Can you work these out from the model? Positions are in its coordinate system, mm. Face numbers are marked on the shaded views. A direction names the side the tool comes from. Round coordinates to 2 decimals unless told otherwise and drop trailing zeros. Write each loop counter-clockwise with the first axis right and the second up, starting at its lowest first coordinate (ties: lowest second). Pieces come first, ordered by that corner, then holes. Notation, with made-up numbers: M 47,8 L 64,8 A28 ccw 64,36 Z; hole C 8,68 d9. An arc over 180 degrees is marked long. Answer in a Markdown table with one row per item. Add a question column.
(1) If I drill on probe 1 along X at (y, z) = (-2.75, 6.2); probe 2 along Z at (x, y) = (29.2, 18.25); probe 3 along X at (y, z) = (36, 5.5), over which ranges is the centre line in solid material (lowest first)?
(2) If we mould it in two halves opening along X, with no side actions, what happens to the marked faces 1, 2, 3 and 4? For each: released by +X, released by -X, zero draft, split by the parting line, or undercut.
(3) I'm going to push flat-ended pins straight in: pin 1 (3.5 mm diameter, centred on x = 32.5, z = 12.5, fed in from -Y); pin 2 (2 mm diameter, centred on x = 5, z = 7, fed in from +Y); pin 3 (3 mm diameter, centred on y = 17.5, z = 10.5, fed in from -X). Where does each tip first touch, or does it pass through?
(4) For the marked faces 5, 6 and 7, which set-ups out of +Z, -Z, +X, -X, +Y, -Y let a thin tool reach every point of the face, with its end or its side?
(5) Suppose I cut it at A-A, the plane y = 18.25. Write out the boundary of the cut face in (x, z), then the cut area to 3 significant figures.
(6) Suppose I cut it at B-B, the plane z = 6.2. Write out the boundary of the cut face in (x, y), then the cut area to 3 significant figures.
(7) Suppose I cut it at D-D, the plane x = 16.5. Write out the boundary of the cut face in (y, z), then the cut area to 3 significant figures.
(8) Suppose I cut it at C-C, the plane z = 2.5. Write out the boundary of the cut face in (x, y).
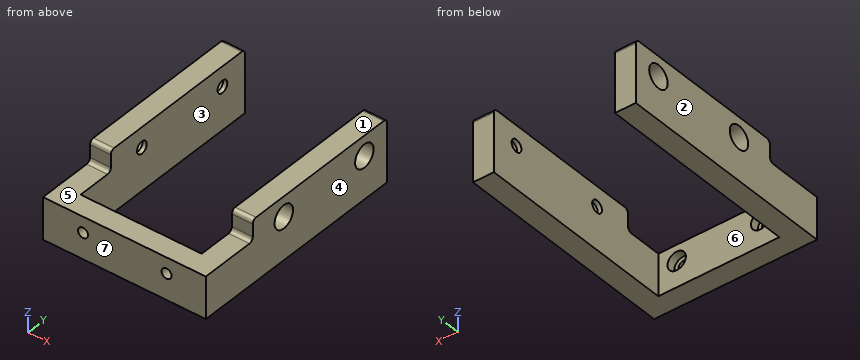
from build123d import *

# Parameters (mm, degrees)
BOSS_EXTRUDE1_DEPTH              = 10
SKETCH2_W                        = 5
SKETCH2_H                        = 40
BOSS_EXTRUDE2_DEPTH              = 5
CBORE_FOR_M2_SHCS1_D             = 2.4
CBORE_FOR_M2_SHCS1_CBORE_D       = 4.4
CBORE_FOR_M2_SHCS1_CBORE_DEPTH   = 2
CBORE_FOR_M2_5_SHCS1_D           = 2.9
CBORE_FOR_M2_5_SHCS1_DEPTH       = 5
CBORE_FOR_M2_5_SHCS1_CBORE_D     = 5.5
CBORE_FOR_M2_5_SHCS1_CBORE_DEPTH = 4
CBORE_FOR_M2_5_SHCS2_D           = 2.9
CBORE_FOR_M2_5_SHCS2_CBORE_D     = 5.5
CBORE_FOR_M2_5_SHCS2_CBORE_DEPTH = 4
FILLET1_R                        = 1


with BuildPart() as part:
    # Sketch1 → Boss-Extrude1 (new body)
    with BuildSketch(Plane.XY):
        Polygon((0, 0), (0, 49), (-5, 49), (-5, -5), (34, -5), (34, 49), (29, 49), (29, 0), align=None)
    extrude(amount=BOSS_EXTRUDE1_DEPTH)

    # Sketch2 → Boss-Extrude2 (add)
    with BuildSketch(Plane.XY.offset(10)):
        with Locations((-2.5, 29)):
            Rectangle(SKETCH2_W, SKETCH2_H)
    boss_extrude2 = extrude(amount=BOSS_EXTRUDE2_DEPTH)

    # Mirror1: Boss-Extrude2 across plane
    add(boss_extrude2.mirror(Plane.ZY.offset(-14.5)))

    # CBORE for M2 SHCS1 (through all)
    with Locations(Plane(origin=(0, 0, 0), x_dir=(1, 0, 0), z_dir=(0, 1, 0))):
        with Locations((24.59562556, -6.2), (4.59562556, -6.2)):
            CounterBoreHole(CBORE_FOR_M2_SHCS1_D / 2, CBORE_FOR_M2_SHCS1_CBORE_D / 2, CBORE_FOR_M2_SHCS1_CBORE_DEPTH)

    # CBORE for M2.5 SHCS1
    with Locations(Plane(origin=(34, 0, 0), x_dir=(0, 0, -1), z_dir=(1, 0, 0))):
        with Locations((-10.2, 42.25), (-10.2, 18.25)):
            CounterBoreHole(CBORE_FOR_M2_5_SHCS1_D / 2, CBORE_FOR_M2_5_SHCS1_CBORE_D / 2, CBORE_FOR_M2_5_SHCS1_CBORE_DEPTH, depth=CBORE_FOR_M2_5_SHCS1_DEPTH)

    # CBORE for M2.5 SHCS2 (through all)
    with Locations(Plane.ZY.offset(5)):
        with Locations((10.2, 42.25), (10.2, 18.25)):
            CounterBoreHole(CBORE_FOR_M2_5_SHCS2_D / 2, CBORE_FOR_M2_5_SHCS2_CBORE_D / 2, CBORE_FOR_M2_5_SHCS2_CBORE_DEPTH)

    # Fillet1
    fillet1_edges = [part.edges().sort_by_distance(p)[0] for p in [
        (-2.5, 9, 10),
        (-2.5, 9, 15),
        (-2.5, 49, 15),
        (31.5, 49, 15),
        (31.5, 9, 15),
        (31.5, 9, 10),
    ]]
    fillet(fillet1_edges, radius=FILLET1_R)


solid = part.part
Calculated:
| question | item | result |
|---|---|---|
| 1 | probe 1 | -5 to 3.4, 5.8 to 23.4, 25.8 to 34 |
| 1 | probe 2 | 0 to 8.75, 11.65 to 15 |
| 1 | probe 3 | -5 to 0, 29 to 34 |
| 2 | face 1 | zero draft |
| 2 | face 2 | released by -X |
| 2 | face 3 | undercut |
| 2 | face 4 | released by +X |
| 3 | pin 1 | y = 8.97 |
| 3 | pin 2 | y = -2 |
| 3 | pin 3 | x = -1 |
| 4 | face 5 | +Z, +X, -X, -Y |
| 4 | face 6 | +Z, -Z, +Y |
| 4 | face 7 | +Z, -Z, +X, -X, -Y |
| 5 | outline | M -5,0 L 0,0 L 0,8.75 L -1,8.75 L -1,7.45 L -5,7.45 Z; M -5,12.95 L -1,12.95 L -1,11.65 L 0,11.65 L 0,15 L -5,15 Z; M 29,0 L 34,0 L 34,7.45 L 30,7.45 L 30,8.75 L 29,8.75 Z; M 29,11.65 L 30,11.65 L 30,12.95 L 34,12.95 L 34,15 L 29,15 Z |
| 5 | area | 100 mm² |
| 6 | outline | M -5,-5 L 3.4,-5 L 3.4,-2 L 2.4,-2 L 2.4,0 L 0,0 L 0,49 L -5,49 Z; M 5.8,-5 L 23.4,-5 L 23.4,-2 L 22.4,-2 L 22.4,0 L 6.8,0 L 6.8,-2 L 5.8,-2 Z; M 25.8,-5 L 34,-5 L 34,49 L 29,49 L 29,0 L 26.8,0 L 26.8,-2 L 25.8,-2 Z |
| 6 | area | 653 mm² |
| 7 | outline | M -5,0 L 0,0 L 0,10 L -5,10 Z |
| 7 | area | 50.0 mm² |
| 8 | outline | M -5,-5 L 34,-5 L 34,49 L 29,49 L 29,0 L 0,0 L 0,49 L -5,49 Z |
